Work out the finished part from the listing and answer in its coordinate system (mm). Face numbers are marked on the shaded views. Give positions to 0.01 mm unless a question says otherwise; leave off trailing zeros. Loops run counter-clockwise (first coordinate to the right, second up) from the corner with the lowest first, then second, coordinate; pieces in that order, holes last. Notation, with made-up numbers: (31.5, -36) - (88.5, -36) arc R19 ccw to (88.5, -26) - close; hole circle Ø3 at (25, 82.25). An arc over 180 degrees is marked (long way). One line per item, written item: value.
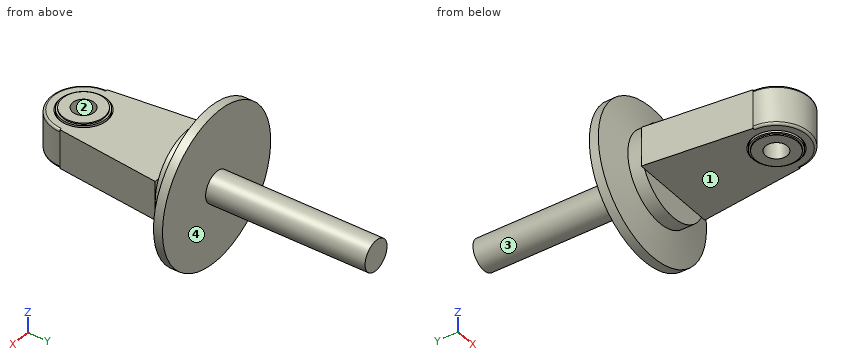
from build123d import *

# Parameters (mm, degrees)
EXTRUDE1_REACH             = 12.1
EXTRUDE1_DIRECTION_2_REACH = 12.1


with BuildPart() as part:
    # Sketch2 → Revolve1 (revolve)
    with BuildSketch(Plane(origin=(0, 0, 0), x_dir=(1, 0, 0), z_dir=(0, 1, 0))):
        with BuildLine():
            Line((5, 10.1), (5, -10.1))
            Line((5, -10.1), (9.6, -10.1))
            Line((9.6, -10.1), (9.6, -9.510239904))
            Line((9.6, -9.510239904), (10.433077185, -9.510239904))
            Line((10.433077185, -9.510239904), (10.433077185, -8.48743323))
            Line((10.433077185, -8.48743323), (10.945643955, -9))
            Line((10.945643955, -9), (14, -9))
            ThreePointArc((14, -9), (14.707106781, -8.707106781), (15, -8))
            Line((15, -8), (15, 8))
            ThreePointArc((15, 8), (14.707106781, 8.707106781), (14, 9))
            Line((14, 9), (10.945643955, 9))
            Line((10.945643955, 9), (10.433077185, 8.48743323))
            Line((10.433077185, 8.48743323), (10.433077185, 9.510239904))
            Line((10.433077185, 9.510239904), (9.6, 9.510239904))
            Line((9.6, 9.510239904), (9.6, 10.1))
            Line((9.6, 10.1), (5, 10.1))
        make_face()
    revolve(axis=Axis((0, 0, -9.945393457), (0, 0, 1)))

    # Extrude1: up to this face of the body (flat: up to its plane)
    extrude1_end = Plane(part.part.faces().sort_by_distance((-11.341623752, 0, 9))[0])
    # Sketch3 → Extrude1 (add, up to the picked face)
    with BuildSketch(Plane.XY, mode=Mode.PRIVATE) as extrude1_sk1:
        with BuildLine():
            Line((-20.25, 47), (-15, 0))
            Line((-15, 0), (-10.945643955, 0))
            ThreePointArc((-10.945643955, 0), (0, 10.945643955), (10.945643955, 0))
            Line((10.945643955, 0), (15, 0))
            Line((15, 0), (20.25, 47))
            Line((20.25, 47), (-20.25, 47))
        make_face()
    extrude1_tool1 = split(extrude(extrude1_sk1.sketch, amount=EXTRUDE1_REACH, mode=Mode.PRIVATE), bisect_by=extrude1_end, keep=Keep.BOTH, mode=Mode.PRIVATE)
    add(extrude1_tool1.solids().sort_by_distance((0, 27.232341, 0))[0])

    # Extrude1 direction 2: up to this face of the body (flat: up to its plane)
    extrude1_direction_2_end = Plane(part.part.faces().sort_by_distance((-13.604020203, 0, -9))[0])
    # Sketch3 → Extrude1 direction 2 (add, up to the picked face)
    with BuildSketch(Plane.XY, mode=Mode.PRIVATE) as extrude1_direction_2_sk1:
        with BuildLine():
            Line((-20.25, 47), (-15, 0))
            Line((-15, 0), (-10.945643955, 0))
            ThreePointArc((-10.945643955, 0), (0, 10.945643955), (10.945643955, 0))
            Line((10.945643955, 0), (15, 0))
            Line((15, 0), (20.25, 47))
            Line((20.25, 47), (-20.25, 47))
        make_face()
    extrude1_direction_2_tool1 = split(extrude(extrude1_direction_2_sk1.sketch, amount=-EXTRUDE1_DIRECTION_2_REACH, mode=Mode.PRIVATE), bisect_by=extrude1_direction_2_end, keep=Keep.BOTH, mode=Mode.PRIVATE)
    add(extrude1_direction_2_tool1.solids().sort_by_distance((0, 27.232341, 0))[0])

    # Sketch7 → Revolve2 (revolve)
    with BuildSketch(Plane.XY):
        Polygon((0, 47), (20.25, 47), (20.25, 53.100825313), (34.5, 56.36235646), (34.5, 60.45), (7, 60.45), (7, 132.908961398), (0, 132.908961398), align=None)
    revolve(axis=Axis((0, 0, 0), (0, 1, 0)))


solid = part.part
1. Section C-C (y = 17) is taken. Write down the section's boundary in (x, z).
Output:
outline: (-16.9, -9) - (16.9, -9) - (16.9, 9) - (-16.9, 9) - close
2. Find the intervals of material crossed by line 1 along Y through (x, z) = (0, 0.75); line 2 along Z through (x, y) = (9, 26); line 3 along Y through (x, z) = (31.5, 14), in increasing order.
Output:
line 1: y = -15 to -5, 5 to 132.91
line 2: z = -9 to 9
line 3: y = 56.36 to 60.45
3. Section A-A (y = 74) is taken. Write down the section's boundary in (x, z).
Output:
outline: circle Ø14 at (0, 0)
4. Flat-ended cylindrical pins translate along their axes: pin 1 Ø5.5 at (x, z) = (1.5, -15.5) entering from -Y; pin 2 Ø16.5 at (x, y) = (4, 2.5) entering from -Z; pin 3 Ø1.1 at (x, z) = (19.5, 5) entering from +Y. Find the tip coordinate at first contact, or state that the pin passes through.
Output:
pin 1: stops at y = 47
pin 2: stops at z = -10.1
pin 3: stops at y = 60.45
5. Section B-B (y = 39) is taken. Write down the section's boundary in (x, z), and give its area (3 significant figures).
Output:
outline: (-19.36, -9) - (19.36, -9) - (19.36, 9) - (-19.36, 9) - close
area: 697 mm²
6. The mould has two halves that part along Y. Classify the marked faces 1, 2, 3 and 4: released by +Y, released by -Y, zero draft, split by the parting line, or undercut.
Output:
face 1: undercut
face 2: undercut
face 3: zero draft
face 4: released by +Y
